Could you check a few things on this model? Use its own coordinates, in mm. Face numbers are marked on the shaded views. A direction names the side the tool comes from. Coordinates: 2 decimals unless noted, no trailing zeros. Loops run counter-clockwise (first coordinate to the right, second up) from the corner with the lowest first, then second, coordinate; pieces in that order, holes last.
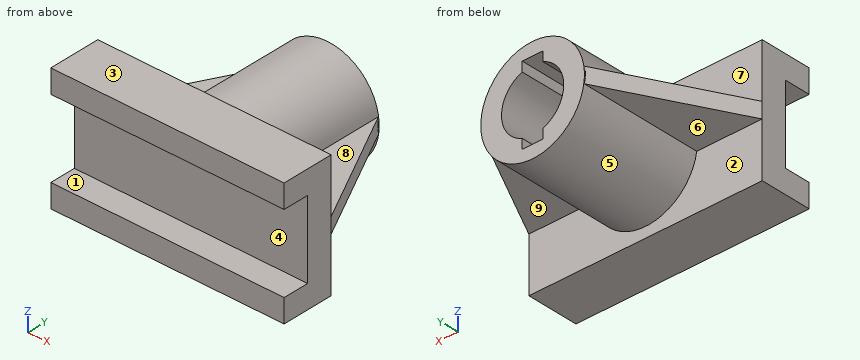
from build123d import *

# Parameters (mm, degrees)
SKETCH1_W               = 90
SKETCH1_H               = 48
BOSS_EXTRUDE1_DEPTH     = 20
SKETCH2_R               = 20
BOSS_EXTRUDE2_DEPTH     = 48
SKETCH3_R               = 12
CUT_EXTRUDE1_DEPTH      = 48
SKETCH4_W               = 8
SKETCH4_H               = 30
CUT_EXTRUDE2_DEPTH      = 48
SKETCH5_W               = 30
SKETCH5_H               = 10
CUT_EXTRUDE4_DEPTH      = 116.325625947
CUT_EXTRUDE4_DEPTH_BACK = 116.325625947
RIB5_REACH              = 87
SKETCH7_WALL_W          = 225.677276384
SKETCH7_WALL_H          = 6


with BuildPart() as part:
    # Sketch1 → Boss-Extrude1 (new body)
    with BuildSketch(Plane(origin=(0, 0, 0), x_dir=(1, 0, 0), z_dir=(0, 1, 0))):
        Rectangle(SKETCH1_W, SKETCH1_H)
    extrude(amount=BOSS_EXTRUDE1_DEPTH)

    # Sketch2 → Boss-Extrude2 (add)
    with BuildSketch(Plane(origin=(0, 20, 0), x_dir=(1, 0, 0), z_dir=(0, 1, 0))):
        with Locations(Location((0, 0, 0), (0, 0, 270))):
            Circle(SKETCH2_R)
    extrude(amount=BOSS_EXTRUDE2_DEPTH)

    # Sketch3 → Cut-Extrude1 (cut)
    with BuildSketch(Plane(origin=(0, 68, 0), x_dir=(1, 0, 0), z_dir=(0, 1, 0))):
        with Locations(Location((0, 0, 0), (0, 0, 270))):
            Circle(SKETCH3_R)
    extrude(amount=-CUT_EXTRUDE1_DEPTH, mode=Mode.SUBTRACT)

    # Sketch4 → Cut-Extrude2 (cut)
    with BuildSketch(Plane(origin=(0, 68, 0), x_dir=(1, 0, 0), z_dir=(0, 1, 0))):
        Rectangle(SKETCH4_W, SKETCH4_H)
    extrude(amount=-CUT_EXTRUDE2_DEPTH, mode=Mode.SUBTRACT)

    # Sketch5 → Cut-Extrude4 (cut, two sides)
    with BuildSketch(Plane.ZY.offset(45)) as cut_extrude4_sk:
        with Locations((0, 5)):
            Rectangle(SKETCH5_W, SKETCH5_H)
    extrude(amount=CUT_EXTRUDE4_DEPTH, mode=Mode.SUBTRACT)
    extrude(cut_extrude4_sk.sketch, amount=-CUT_EXTRUDE4_DEPTH_BACK, mode=Mode.SUBTRACT)

    # Sketch7 wall → Rib5 (add, up to next)
    with BuildSketch(Plane(origin=(32.5, 43.75, 0), x_dir=(0.465746432833, -0.884918222382, 0), z_dir=(0.884918222382, 0.465746432833, 0)), mode=Mode.PRIVATE) as rib5_sk1:
        Rectangle(SKETCH7_WALL_W, SKETCH7_WALL_H)
    rib5_tool1 = extrude(rib5_sk1.sketch, amount=-RIB5_REACH, mode=Mode.PRIVATE) - part.part
    add(rib5_tool1.solids().sort_by_distance((32.5, 43.75, 0))[0])

    # Mirror1: part across plane


with BuildPart() as part_1:
    add(part.part)
    add(part.part.mirror(Plane(origin=(0, 0, 0), x_dir=(0, 0, 1), z_dir=(1, 0, 0))))


solid = part_1.part
(1) Imagine slicing it at B-B, the plane x = 31.5. Write out the boundary of the cut face in (y, z).
Answers:
outline: (0, -24) - (20, -24) - (20, -3) - (45.65, -3) - (45.65, 3) - (20, 3) - (20, 24) - (0, 24) - (0, 15) - (10, 15) - (10, -15) - (0, -15) - close
(2) We'd pull the mould along Z, two halves only. Please class the marked faces 1, 2, 3 and 4: +Z half, -Z half, draft (parallel to the pull), parting line (faces both ways), or undercut.
Answers:
face 1: undercut
face 2: draft
face 3: +Z half
face 4: undercut
(3) Which directions (+Z, -Z, +X, -X, +Y, -Y) give clear straight access to the entire face, cutting with the end or side of a thin tool? Please do the marked faces 5, 6, 7, 8 and 9.
Answers:
face 5: +Y
face 6: -Z, -X, +Y
face 7: +Z, +Y
face 8: +Z, +X, +Y
face 9: -Z, +X, +Y
(4) For pin 1 (2 mm diameter, centred on x = 26.5, z = -13.5, fed in from -Y); pin 2 (1.8 mm diameter, centred on y = 48, z = -14, fed in from +X); pin 3 (2.5 mm diameter, centred on x = 1, y = 35.5, fed in from +Z), each with a flat end and sliding along its axis, tell me the tip position at first contact or that it passes through.
Answers:
pin 1: stops at y = 10
pin 2: stops at x = 15.11
pin 3: stops at z = 20
(5) Imagine slicing it at D-D, the plane z = -9. Write out the boundary of the cut face in (x, y), and give its area (3 significant figures).
Answers:
outline: (-45, 10) - (45, 10) - (45, 20) - (17.86, 20) - (17.86, 68) - (7.94, 68) - (7.94, 20) - (-7.94, 20) - (-7.94, 68) - (-17.86, 68) - (-17.86, 20) - (-45, 20) - close
area: 1,850 mm2
(6) Imagine slicing it at C-C, the plane y = 31. Write out the boundary of the cut face in (x, z), and give its area (3 significant figures).
Answers:
outline: (-39.21, -3) - (-19.77, -3) arc R20 ccw to (19.77, -3) - (39.21, -3) - (39.21, 3) - (19.77, 3) arc R20 ccw to (-19.77, 3) - (-39.21, 3) - close; hole (-4, -15) - (4, -15) - (4, -11.31) arc R12 ccw to (4, 11.31) - (4, 15) - (-4, 15) - (-4, 11.31) arc R12 ccw to (-4, -11.31) - close
area: 984 mm2
(7) Imagine slicing it at A-A, the plane y = 7.5. Write out the boundary of the cut face in (x, z).
Answers:
outline: (-45, -24) - (45, -24) - (45, -15) - (-45, -15) - close; (-45, 15) - (45, 15) - (45, 24) - (-45, 24) - close
(8) I need wall thicknesses on probe 1 along Z at (x, y) = (-21.5, 6.5); probe 2 along Y at (x, z) = (29, 13.5); probe 3 along Z at (x, y) = (26.5, 37). Which ranges of each line are inside material? Lowest first, please.
Answers:
probe 1: z = -24 to -15, 15 to 24
probe 2: y = 10 to 20
probe 3: z = -3 to 3
